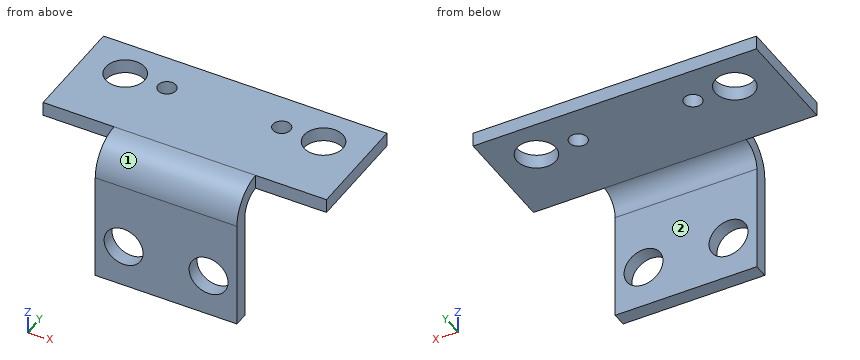
from build123d import *

# Parameters (mm, degrees)
SKETCH_1_W                       = 20
SKETCH_1_H                       = 20
SM_BASE_FLANGE_1_DEPTH           = 2
SM_EDGE_FLANGE_1_STRIP_W         = 13.4732
SM_EDGE_FLANGE_1_STRIP_H         = 2
SM_EDGE_FLANGE_1_STRIP_CUT_DEPTH = 20
SM_EDGE_FLANGE_1_DEPTH           = 20
SM_EDGE_FLANGE_1_PROFILE_W       = 40
SM_EDGE_FLANGE_1_PROFILE_H       = 15.2634
SM_EDGE_FLANGE_1_FLAT_DEPTH      = 2
SKETCH_9_R                       = 2.75
SKETCH_9_R_2                     = 1.25
CUT_EXTRUDE_1_DEPTH              = 10
SKETCH_10_R                      = 2.75
CUT_EXTRUDE_2_DEPTH              = 10


# Sheet-metal steps are written as plain solids
with BuildPart() as part:
    # Sketch 1 → 基体-法兰1 (new body)
    with BuildSketch(Plane(origin=(0, 0, 0), x_dir=(1, 0, 0), z_dir=(0, 1, 0))):
        Rectangle(SKETCH_1_W, SKETCH_1_H)
    extrude(amount=-SM_BASE_FLANGE_1_DEPTH)

    # 边线-法兰1 strip (across the edge) → 边线-法兰1 strip cut (cut)
    with BuildSketch(Plane(origin=(-10, 0, 10), x_dir=(0, 0, -1), z_dir=(1, 0, 0))):
        with Locations((-2, -1)):
            Rectangle(SM_EDGE_FLANGE_1_STRIP_W, SM_EDGE_FLANGE_1_STRIP_H)
    extrude(amount=SM_EDGE_FLANGE_1_STRIP_CUT_DEPTH, mode=Mode.SUBTRACT)

    # 边线-法兰1 bend section (across the edge) → 边线-法兰1 (add)
    with BuildSketch(Plane(origin=(-10, 0, 10), x_dir=(0, 0, -1), z_dir=(1, 0, 0))):
        with BuildLine():
            Line((0, 2.7366), (2, 2.7366))
            ThreePointArc((2, 2.7366), (2.801531583, 0.801531583), (4.7366, 0))
            Line((4.7366, 0), (4.7366, -2))
            ThreePointArc((4.7366, -2), (1.38731802, -0.61268198), (0, 2.7366))
        make_face()
    extrude(amount=SM_EDGE_FLANGE_1_DEPTH)

    # 边线-法兰1 profile (on flange) → 边线-法兰1 flat (add)
    with BuildSketch(Plane(origin=(0, 0, 10), x_dir=(-1, 0, 0), z_dir=(0, 0, -1))):
        with Locations((0, 10.3683)):
            Rectangle(SM_EDGE_FLANGE_1_PROFILE_W, SM_EDGE_FLANGE_1_PROFILE_H)
    extrude(amount=SM_EDGE_FLANGE_1_FLAT_DEPTH)

    # 草图9 → 切除-拉伸1 (cut)
    with BuildSketch(Plane.XY.offset(10)):
        with Locations((14, 12.7366)):
            Circle(SKETCH_9_R)
        with Locations((8.1, 12.7366)):
            Circle(SKETCH_9_R_2)
        with Locations(Location((-8.1, 12.7366, 0), (0, 0, 270))):
            Circle(SKETCH_9_R_2)
        with Locations(Location((-14, 12.7366, 0), (0, 0, 270))):
            Circle(SKETCH_9_R)
    extrude(amount=-CUT_EXTRUDE_1_DEPTH, mode=Mode.SUBTRACT)

    # 草图10 → 切除-拉伸2 (cut)
    with BuildSketch(Plane.XZ.offset(2)):
        with Locations(Location((6, -4, 0), (0, 0, 270))):
            Circle(SKETCH_10_R)
        with Locations(Location((-6, -4, 0), (0, 0, 270))):
            Circle(SKETCH_10_R)
    extrude(amount=-CUT_EXTRUDE_2_DEPTH, mode=Mode.SUBTRACT)


solid = part.part
The model under review builds one solid part; all positions refer to its coordinate system, in mm. Face numbers are marked on the shaded views. A direction names the side the tool comes from. Give positions to 0.01 mm unless a question says otherwise; leave off trailing zeros. Write each loop counter-clockwise with the first axis right and the second up, starting at its lowest first coordinate (ties: lowest second). Pieces come first, ordered by that corner, then holes.
1. Tool access review of the marked faces 1 and 2: name each direction out of +Z, -Z, +X, -X, +Y, -Y from which nothing blocks a thin tool from reaching the whole face with its end or side.
2. Add section A-A, the plane z = -4. Write out the cut boundary in (x, y), plus the area to 3 significant figures.
3. Add section C-C, the plane x = -2.5. Write out the cut boundary in (y, z).
4. Wall thickness on L1, parallel to X at y = -0.95, z = -4; L2, parallel to Z at x = -2.5, y = 2.75; L3, parallel to Y at x = -9, z = -2.25: over which ranges is each line inside the solid? List them lowest first.
5. Add section B-B, the plane x = 6. Write out the cut boundary in (y, z).
6. Add section D-D, the plane y = 16.25. Write out the cut boundary in (x, z), plus the area to 3 significant figures.
7. For P1, Ø2, axis at x = -14, z = 9, coming from the -Y side; P2, Ø8, axis at x = 3, y = 6.5, coming from the -Z side; P3, Ø9, axis at x = 6, z = -4, coming from the +Y side; P4, Ø2, axis at x = 8.1, y = 12.74, coming from the -Z side, all flat-tipped, find the tip position at first contact; note any pin that passes through.
Worked answers:
1. face 1: +Z, +X, -X, -Y
1. face 2: -Z, +X, -X, +Y
2. outline: (-10, -2) - (-8.75, -2) - (-8.75, 0) - (-10, 0) - close; (-3.25, -2) - (3.25, -2) - (3.25, 0) - (-3.25, 0) - close; (8.75, -2) - (10, -2) - (10, 0) - (8.75, 0) - close
2. area: 18.0 mm2
3. outline: (-2, -10) - (0, -10) - (0, 5.26) arc R2.74 cw to (2.74, 8) - (18, 8) - (18, 10) - (2.74, 10) arc R4.74 ccw to (-2, 5.26) - close
4. L1: x = -10 to -8.75, -3.25 to 3.25, 8.75 to 10
4. L2: z = 8 to 10
4. L3: y = -2 to 0
5. outline: (-2, -10) - (0, -10) - (0, -6.75) - (-2, -6.75) - close; (-2, -1.25) - (0, -1.25) - (0, 5.26) arc R2.74 cw to (2.74, 8) - (18, 8) - (18, 10) - (2.74, 10) arc R4.74 ccw to (-2, 5.26) - close
6. outline: (-20, 8) - (20, 8) - (20, 10) - (-20, 10) - close
6. area: 80.0 mm2
7. P1: stops at y = 2.74
7. P2: stops at z = 7.99
7. P3: stops at y = 0
7. P4: passes through
